Geometry: final body of the model. Coordinates: model frame, mm. A direction names the side the tool comes from. Coordinates: 2 decimals unless noted, no trailing zeros. Order: outer loops, then holes, each group sorted by start corner. A loop starts at its lowest first (then second) coordinate and runs counter-clockwise, first axis right, second up. Notation, with made-up numbers: M -13.5,15 L 43.5,15 A21 cw 43.5,36 Z; hole C 30,15.5 d2. An arc over 180 degrees is marked long. Use CSV: the item, a comma, the result in double quotes. Start each with the question number.
Q1. Mould query, pull axis Y, two halves, no side actions, for faces 1 (the face through (0.18, 19.76, -12.77)), 2 (the face through (10, 3, -4)), 3 (the face through (-12.2, 12, 0)). Classes: +Y half, -Y half, draft (parallel to the pull), parting line (faces both ways), or undercut.
Q2. Ray query, probe 1 along Z at (x, y) = (5.75, 17.75); probe 2 along Z at (x, y) = (-6.5, 2.25). Return the intervals inside material, ascending.
Q3. Section query B-B, the plane x = 8.75. State how many separate pieces and enclosed holes the cut face has, and give its area (3 significant figures).
Q4. Section query A-A, the plane y = 11.5. Output: boundary loops of the cut face in (x, z), and give its area (3 significant figures).
Q5. Access query for faces 4 (the face through (-5, 0, 9)), 5 (the face through (4, 3, -10)), 6 (the face through (0, 12, -12.2)). Directions: +Z, -Z, +X, -X, +Y, -Y. A direction counts if a zero-diameter tool reaches every point of the face in a straight line with its end or side. Return the directions, or none.
Q6. First-contact query: P1, Ø3, axis at x = -6.5, z = 6.5, coming from the -Y side. Flat tip, straight axial feed; report the tip coordinate or a pass-through.
from build123d import *

# Parameters (mm, degrees)
SKETCH1_W           = 26
SKETCH1_H           = 26
BOSS_EXTRUDE1_DEPTH = 8
SKETCH24_W          = 26
SKETCH24_H          = 26
SKETCH24_W_2        = 24.4
SKETCH24_H_2        = 24.4
BOSS_EXTRUDE5_DEPTH = 11.6
SKETCH27_W          = 26
SKETCH27_H          = 26
BOSS_EXTRUDE7_DEPTH = 0.4
FILLET2_R           = 0.8


with BuildPart() as part:
    # Sketch1 → Boss-Extrude1 (new body)
    with BuildSketch(Plane(origin=(0, 0, 0), x_dir=(1, 0, 0), z_dir=(0, 1, 0))):
        Rectangle(SKETCH1_W, SKETCH1_H)
        with BuildLine():
            Line((-4, 7.214142843), (-4, 12.2))
            Line((-4, 12.2), (4, 12.2))
            Line((4, 12.2), (4, 7.214142843))
            ThreePointArc((4, 7.214142843), (8.338477631, 8.338477631), (7.214142843, 4))
            Line((7.214142843, 4), (12.2, 4))
            Line((12.2, 4), (12.2, -4))
            Line((12.2, -4), (7.214142843, -4))
            ThreePointArc((7.214142843, -4), (8.338477631, -8.338477631), (4, -7.214142843))
            Line((4, -7.214142843), (4, -12.2))
            Line((4, -12.2), (-4, -12.2))
            Line((-4, -12.2), (-4, -7.214142843))
            ThreePointArc((-4, -7.214142843), (-8.338477631, -8.338477631), (-7.214142843, -4))
            Line((-7.214142843, -4), (-12.2, -4))
            Line((-12.2, -4), (-12.2, 4))
            Line((-12.2, 4), (-7.214142843, 4))
            ThreePointArc((-7.214142843, 4), (-8.338477631, 8.338477631), (-4, 7.214142843))
        make_face(mode=Mode.SUBTRACT)
    extrude(amount=BOSS_EXTRUDE1_DEPTH)

    # Sketch21 → Cut-Loft5 section 0
    with BuildSketch(Plane(origin=(0, 1, 0), x_dir=(1, 0, 0), z_dir=(0, 1, 0))):
        with BuildLine():
            Line((-7.5, -7.5), (7.5, -7.5))
            Line((7.5, -7.5), (7.5, 7.5))
            Line((7.5, 7.5), (-7.5, 7.5))
            Line((-7.5, 7.5), (-7.5, -7.5))
        make_face()
    # Sketch22 → Cut-Loft5 section 1
    with BuildSketch(Plane(origin=(0, 8, 0), x_dir=(1, 0, 0), z_dir=(0, 1, 0))):
        with BuildLine():
            Line((-12.2, -12.2), (12.2, -12.2))
            Line((12.2, -12.2), (12.2, 12.2))
            Line((12.2, 12.2), (-12.2, 12.2))
            Line((-12.2, 12.2), (-12.2, -12.2))
        make_face()
    loft(mode=Mode.SUBTRACT)

    # Sketch24 → Boss-Extrude5 (add)
    with BuildSketch(Plane(origin=(0, 8, 0), x_dir=(1, 0, 0), z_dir=(0, 1, 0))):
        Rectangle(SKETCH24_W, SKETCH24_H)
        Rectangle(SKETCH24_W_2, SKETCH24_H_2, mode=Mode.SUBTRACT)
    extrude(amount=BOSS_EXTRUDE5_DEPTH)

    # Sketch27 → Boss-Extrude7 (add)
    with BuildSketch(Plane(origin=(0, 19.6, 0), x_dir=(1, 0, 0), z_dir=(0, 1, 0))):
        Rectangle(SKETCH27_W, SKETCH27_H)
    extrude(amount=BOSS_EXTRUDE7_DEPTH)

    # Fillet2
    fillet2_edges = [part.edges().sort_by_distance(p)[0] for p in [
        (13, 20, 0),
        (0, 20, -13),
        (-13, 20, 0),
        (0, 20, 13),
    ]]
    fillet(fillet2_edges, radius=FILLET2_R)


solid = part.part
Responses:
1,face 1,"+Y half"
1,face 2,"draft"
1,face 3,"undercut"
2,probe 1,"z = -13 to -12.2, 12.2 to 13"
2,probe 2,"z = -13 to -9.1, 9.1 to 13"
3,separate pieces,"3"
3,enclosed holes,"0"
3,area,"91.2 mm²"
4,outline,"M -13,-13 L 13,-13 L 13,13 L -13,13 Z; hole M -12.2,-12.2 L 12.2,-12.2 L 12.2,12.2 L -12.2,12.2 Z"
4,area,"80.6 mm²"
5,face 4,"+Z, -Z, +X, -X, -Y"
5,face 5,"-Y"
5,face 6,"none"
6,P1,"stops at y = 19.6"
